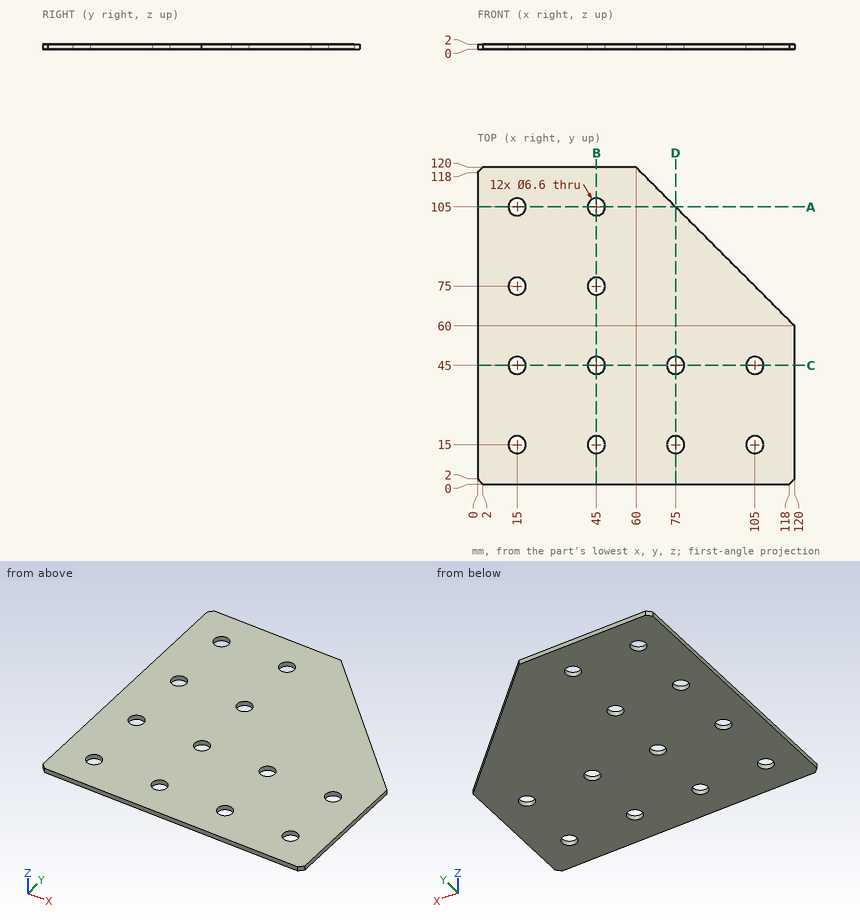
Input: dimensioned drawing with shaded views. Units: mm. Origin: part minimum x, y, z. Round coordinates to 2 decimals unless told otherwise and drop trailing zeros. Loops run counter-clockwise (first coordinate to the right, second up) from the corner with the lowest first, then second, coordinate; pieces in that order, holes last. Notation, with made-up numbers: (-11, -3.5) -> (1, -3.5) arc R22 cw to (1, 6.5) -> close; hole circle Ø6 at (-35.75, 3). An arc over 180 degrees is marked (long way). Answer as a JSON object with one key per item and string values. Group by question number.
Q1. Ray query, line 1 (Y direction, x = 45, z = 1.5); line 2 (Y direction, x = 105, z = 1.45). Return the intervals inside material, ascending. Write a range as from..to.
Q2. Section query D-D (x = 75). Output: boundary loops of the cut face in (y, z), plus the area to 3 significant figures.
Q3. Section query A-A (y = 105). Output: boundary loops of the cut face in (x, z).
Q4. Section query B-B (x = 45). Output: boundary loops of the cut face in (y, z).
Completed:
{
 "1": {"line 1": "0..11.7, 18.3..41.7, 48.3..71.7, 78.3..101.7, 108.3..120", "line 2": "0..11.7, 18.3..41.7, 48.3..75"},
 "2": {"outline": "(0, 0) -> (11.7, 0) -> (11.7, 2) -> (0, 2) -> close; (18.3, 0) -> (41.7, 0) -> (41.7, 2) -> (18.3, 2) -> close; (48.3, 0) -> (105, 0) -> (105, 2) -> (48.3, 2) -> close", "area": "184 mm²"},
 "3": {"outline": "(0, 0) -> (11.7, 0) -> (11.7, 2) -> (0, 2) -> close; (18.3, 0) -> (41.7, 0) -> (41.7, 2) -> (18.3, 2) -> close; (48.3, 0) -> (75, 0) -> (75, 2) -> (48.3, 2) -> close"},
 "4": {"outline": "(0, 0) -> (11.7, 0) -> (11.7, 2) -> (0, 2) -> close; (18.3, 0) -> (41.7, 0) -> (41.7, 2) -> (18.3, 2) -> close; (48.3, 0) -> (71.7, 0) -> (71.7, 2) -> (48.3, 2) -> close; (78.3, 0) -> (101.7, 0) -> (101.7, 2) -> (78.3, 2) -> close; (108.3, 0) -> (120, 0) -> (120, 2) -> (108.3, 2) -> close"}
}
